Source: CAD feature listing. Evaluate the final solid. Frame: model axes, mm. A direction names the side the tool comes from. Round coordinates to 2 decimals unless told otherwise and drop trailing zeros. Write each loop counter-clockwise with the first axis right and the second up, starting at its lowest first coordinate (ties: lowest second). Pieces come first, ordered by that corner, then holes. Notation, with made-up numbers: M 25.25,-27.75 L 51.25,-27.75 A19 ccw 51.25,-23.75 Z; hole C 3,32 d11. An arc over 180 degrees is marked long. Answer in a Markdown table with one row per item.
Autodesk Inventor part; units mm, degrees
ref_plane "YZ Plane" through (0, 0, 0) normal (1, 0, 0) x (0, 1, 0)
ref_plane "XZ Plane" through (0, 0, 0) normal (0, 1, 0) x (-1, 0, 0)
ref_plane "XY Plane" through (0, 0, 0) normal (0, 0, 1) x (1, 0, 0)
sketch "Sketch1" plane through (0, 0, 0) normal (0, 0, 1) x (1, 0, 0)
  circle A0 centre (0, 0) radius 15
  dimension "d0" = 30
extrude "Extrusion1" add sketch "Sketch1" along normal blind 10
sketch "Sketch2" plane through (0, 0, 10) normal (0, 0, 1) x (1, 0, 0)
  circle A0 centre (0, 0) radius 2
  dimension "d3" = 4
extrude "Extrusion2" cut sketch "Sketch2" against normal blind 1.5
sketch "Sketch3" plane through (0, 0, 0) normal (0, 0, -1) x (-1, 0, 0)
  circle A0 centre (0, -11.4062) radius 1.5
  point P0 (0, 0)
  dimension "d6" = 3
extrude "Extrusion3" add sketch "Sketch3" along normal blind 8
properties material "Water"
Q1. Contact query for flat-ended pins moving along their axis: pin 1 Ø8 at (x, z) = (3.5, -4.5) entering from +Y; pin 2 Ø2 at (x, y) = (-8.5, -8) entering from -Z; pin 3 Ø3.5 at (x, y) = (0, 0) entering from +Z. Output: stop coordinate, or through.
Solutions:
| item | result |
|---|---|
| pin 1 | stops at y = -9.91 |
| pin 2 | stops at z = 0 |
| pin 3 | stops at z = 8.5 |
Q2. Section B-B (x = 0). Return loops of the section in (y, z), and give its area (3 significant figures).
Solutions:
| item | result |
|---|---|
| outline | M -15,0 L -12.91,0 L -12.91,-8 L -9.91,-8 L -9.91,0 L 15,0 L 15,10 L 2,10 L 2,8.5 L -2,8.5 L -2,10 L -15,10 Z |
| area | 318 mm2 |
Q3. Access query for faces 4 (the flat face through (0, 0, 8.5)), 5 (the flat face through (0, -3, 10)). Directions: +Z, -Z, +X, -X, +Y, -Y. A direction counts if a zero-diameter tool reaches every point of the face in a straight line with its end or side. Return the directions, or none.
Solutions:
| item | result |
|---|---|
| face 4 | +Z |
| face 5 | +Z, +X, -X, +Y, -Y |
Q4. Material intervals for probe 1 along Y at (x, z) = (0, 9.6); probe 2 along Z at (x, y) = (12.5, 7.75); probe 3 along X at (y, z) = (-0.5, 4.75), sorted ascending.
Solutions:
| item | result |
|---|---|
| probe 1 | y = -15 to -2, 2 to 15 |
| probe 2 | z = 0 to 10 |
| probe 3 | x = -14.99 to 14.99 |
Q5. Section D-D (y = -9). Return loops of the section in (x, z).
Solutions:
| item | result |
|---|---|
| outline | M -12,0 L 12,0 L 12,10 L -12,10 Z |
Q6. Pull-direction query (Y, two-part tool) for faces 1 (the cylindrical face through (0, -2, 9)), 2 (the cylindrical face through (0.325, -9.942, -3.944)), 3 (the flat face through (0, -11, -8)); classes: pulls with the +Y half, pulls with the -Y half, needs draft (parallel to the pull), parting line crosses it, or undercut.
Solutions:
| item | result |
|---|---|
| face 1 | undercut |
| face 2 | parting line crosses it |
| face 3 | needs draft |
Q7. Section C-C (z = 1.75). Return loops of the section in (x, y).
Solutions:
| item | result |
|---|---|
| outline | C 0,0 d30 |
Q8. Section A-A (y = 0). Return loops of the section in (x, z), and give its area (3 significant figures).
Solutions:
| item | result |
|---|---|
| outline | M -15,0 L 15,0 L 15,10 L 2,10 L 2,8.5 L -2,8.5 L -2,10 L -15,10 Z |
| area | 294 mm2 |
